Work out the finished part from the listing and answer in its coordinate system (mm). Face numbers are marked on the shaded views. A direction names the side the tool comes from. Round coordinates to 2 decimals unless told otherwise and drop trailing zeros. Loops run counter-clockwise (first coordinate to the right, second up) from the corner with the lowest first, then second, coordinate; pieces in that order, holes last. Notation, with made-up numbers: (5.25, 79.5) -> (57.25, 79.5) arc R24 cw to (57.25, 106.5) -> close; hole circle Ø1 at (66, -20). An arc over 180 degrees is marked (long way). Use CSV: the item, a comma, the result in double quotes. Start each with the question number.
from build123d import *

# Parameters (mm, degrees)
SKETCH1_R           = 11.2
BOSS_EXTRUDE1_DEPTH = 204.313708212
CUT_EXTRUDE1_DEPTH  = 236.982


with BuildPart() as part:
    # Sketch1 → Boss-Extrude1 (new body)
    with BuildSketch(Plane.XY):
        with BuildLine():
            Line((-25.4, -67.479999962), (-25.4, 36.365))
            ThreePointArc((-25.4, 36.365), (-23.726115254, 40.406115254), (-19.685, 42.08))
            Line((-19.685, 42.08), (32.385, 42.08))
            ThreePointArc((32.385, 42.08), (36.426115254, 40.406115254), (38.1, 36.365))
            Line((38.1, 36.365), (38.1, 35.095))
            ThreePointArc((38.1, 35.095), (36.426115254, 31.053884746), (32.385, 29.38))
            Line((32.385, 29.38), (-9.652, 29.38))
            ThreePointArc((-9.652, 29.38), (-11.807261469, 28.487261469), (-12.7, 26.332))
            Line((-12.7, 26.332), (-12.7, 22.503))
            ThreePointArc((-12.7, 22.503), (-11.807261469, 20.347738531), (-9.652, 19.455))
            Line((-9.652, 19.455), (0, 19.455))
            Line((0, 19.455), (13.74, 19.455))
            ThreePointArc((13.74, 19.455), (17.781115254, 17.781115254), (19.455, 13.74))
            Line((19.455, 13.74), (19.455, 0))
            Line((19.455, 0), (19.455, -13.74))
            ThreePointArc((19.455, -13.74), (17.781115254, -17.781115254), (13.74, -19.455))
            Line((13.74, -19.455), (0, -19.455))
            Line((0, -19.455), (-9.652, -19.455))
            ThreePointArc((-9.652, -19.455), (-11.807261469, -20.347738531), (-12.7, -22.503))
            Line((-12.7, -22.503), (-12.7, -26.331999962))
            ThreePointArc((-12.7, -26.331999962), (-11.807261469, -28.487261431), (-9.652, -29.379999962))
            Line((-9.652, -29.379999962), (32.385, -29.379999962))
            ThreePointArc((32.385, -29.379999962), (36.426115254, -31.053884708), (38.1, -35.094999962))
            Line((38.1, -35.094999962), (38.1, -67.479999962))
            ThreePointArc((38.1, -67.479999962), (36.240128061, -71.970128023), (31.75, -73.829999962))
            Line((31.75, -73.829999962), (-19.05, -73.829999962))
            ThreePointArc((-19.05, -73.829999962), (-23.540128061, -71.970128023), (-25.4, -67.479999962))
        make_face()
        Circle(SKETCH1_R, mode=Mode.SUBTRACT)
    extrude(amount=BOSS_EXTRUDE1_DEPTH)

    # Sketch2 → Cut-Extrude1 (cut)
    with BuildSketch(Plane.XY.offset(204.313708212)):
        with BuildLine():
            ThreePointArc((32.385, 29.38), (36.426115254, 31.053884746), (38.1, 35.095))
            Line((38.1, 35.095), (38.1, 36.365))
            ThreePointArc((38.1, 36.365), (36.426115254, 40.406115254), (32.385, 42.08))
            Line((32.385, 42.08), (19.455, 42.08))
            Line((19.455, 42.08), (19.455, 29.38))
            Line((19.455, 29.38), (32.385, 29.38))
        make_face()
        with BuildLine():
            Line((-9.652, 29.38), (19.455, 29.38))
            Line((19.455, 29.38), (19.455, 42.08))
            Line((19.455, 42.08), (-12.7, 42.08))
            Line((-12.7, 42.08), (-12.7, 26.332))
            ThreePointArc((-12.7, 26.332), (-11.807261469, 28.487261469), (-9.652, 29.38))
        make_face()
        with BuildLine():
            Line((19.455, 13.74), (19.455, -13.74))
            Line((19.455, -13.74), (38.1, -13.74))
            Line((38.1, -13.74), (38.1, 35.095))
            ThreePointArc((38.1, 35.095), (36.426115254, 31.053884746), (32.385, 29.38))
            Line((32.385, 29.38), (19.455, 29.38))
            Line((19.455, 29.38), (19.455, 22.503))
            Line((19.455, 22.503), (19.455, 13.74))
        make_face()
        with BuildLine():
            ThreePointArc((32.385, 42.08), (36.426115254, 40.406115254), (38.1, 36.365))
            Line((38.1, 36.365), (38.1, 42.08))
            Line((38.1, 42.08), (32.385, 42.08))
        make_face()
        with BuildLine():
            Line((-12.7, 22.503), (19.455, 22.503))
            Line((19.455, 22.503), (19.455, 29.38))
            Line((19.455, 29.38), (-9.652, 29.38))
            ThreePointArc((-9.652, 29.38), (-11.807261469, 28.487261469), (-12.7, 26.332))
            Line((-12.7, 26.332), (-12.7, 22.503))
        make_face()
    extrude(amount=-CUT_EXTRUDE1_DEPTH, mode=Mode.SUBTRACT)


solid = part.part
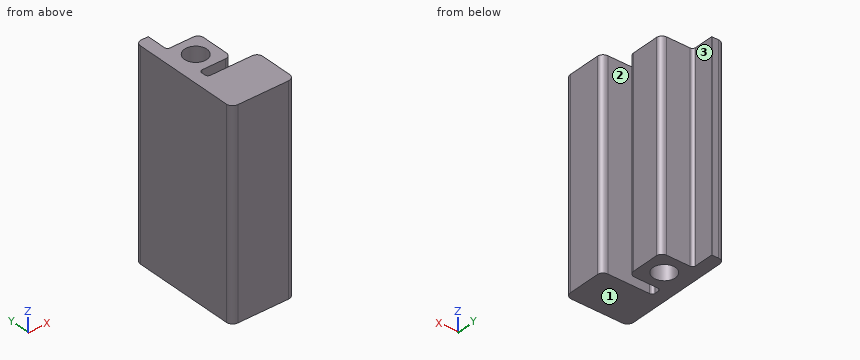
Q1. Which of the six approach directions +Z, -Z, +X, -X, +Y, -Y give full straight-line access (tool end or side, diameter ignored) to the marked faces 1, 2 and 3?
Q2. Each of these flat-tipped pins is pushed along its axis until it touches: pin 1 (2 mm diameter, centred on y = -26.5, z = 110, fed in from +X); pin 2 (10 mm diameter, centred on y = 29, z = 52.5, fed in from +X); pin 3 (12 mm diameter, centred on y = -3.5, z = 165, fed in from +X) (3 decimals); pin 4 (18 mm diameter, centred on x = 0, y = 0, fed in from -Z). Where does it stop, or does it pass through?
Q3. Straight lines are drawn through the part: line 1 (Y direction, x = 0, z = 78) (3 decimals); line 2 (Y direction, x = 2.5, z = 184.5) (3 decimals); line 3 (Y direction, x = 13.5, z = 20.5) (3 decimals). For each, find the intervals that lie inside material, in ascending order. Write a range as from..to.
Q4. Section C-C, the plane z = 187.5 is taken. Write down the section's boundary in (x, y) (3 decimals).
Q5. Section A-A, the plane x = 0 is taken. Write down the section's boundary in (y, z) (3 decimals), and give its area (3 significant figures).
Q6. Section B-B, the plane y = 0 is taken. Write down the section's boundary in (x, z) (3 decimals).
Report:
1,face 1,"-Z, +X, -X, +Y, -Y"
1,face 2,"+Z, -Z, +X"
1,face 3,"+Z, -Z, +X, +Y"
2,pin 1,"stops at x = -12.47"
2,pin 2,"stops at x = -12.7"
2,pin 3,"stops at x = 19.455"
2,pin 4,"passes through"
3,line 1,"y = -73.83..-29.38, -19.455..-11.2, 11.2..19.455"
3,line 2,"y = -73.83..-29.38, -19.455..-10.917, 10.917..19.455"
3,line 3,"y = -73.83..-29.38, -19.455..19.455"
4,outline,"(-25.4, -67.48) arc R6.35 ccw to (-19.05, -73.83) -> (31.75, -73.83) arc R6.35 ccw to (38.1, -67.48) -> (38.1, -35.095) arc R5.715 ccw to (32.385, -29.38) -> (-9.652, -29.38) arc R3.048 cw to (-12.7, -26.332) -> (-12.7, -22.503) arc R3.048 cw to (-9.652, -19.455) -> (13.74, -19.455) arc R5.715 ccw to (19.455, -13.74) -> (19.455, 13.74) arc R5.715 ccw to (13.74, 19.455) -> (-9.652, 19.455) arc R3.048 cw to (-12.7, 22.503) -> (-12.7, 42.08) -> (-19.685, 42.08) arc R5.715 ccw to (-25.4, 36.365) -> close; hole circle Ø22.4 at (0, 0)"
5,outline,"(-73.83, 0) -> (-29.38, 0) -> (-29.38, 204.314) -> (-73.83, 204.314) -> close; (-19.455, 0) -> (-11.2, 0) -> (-11.2, 204.314) -> (-19.455, 204.314) -> close; (11.2, 0) -> (19.455, 0) -> (19.455, 204.314) -> (11.2, 204.314) -> close"
5,area,"12,500 mm²"
6,outline,"(-25.4, 0) -> (-11.2, 0) -> (-11.2, 204.314) -> (-25.4, 204.314) -> close; (11.2, 0) -> (19.455, 0) -> (19.455, 204.314) -> (11.2, 204.314) -> close"
